Solid Edge part; units mm, degrees
sketch "Sketch1" plane through (0, 0, 0) normal (0, 0, 1) x (1, 0, 0)
  circle A0 centre (0, 0) radius 25.5
extrude "Ajout_matière_1" add sketch "Sketch1" along normal mid plane 71
sketch "Sketch2" plane through (0, 0, 35.5) normal (0, 0, 1) x (1, 0, 0)
  circle A0 centre (0, 0) radius 13
  circle A1 centre (0, 0) radius 5.5
extrude "Ajout_matière_2" add sketch "Sketch2" along normal blind 6
sketch "Sketch3" plane through (0, 0, 35.5) normal (0, 0, 1) x (1, 0, 0)
  circle A0 centre (20.5, 0) radius 2
extrude "Ajout_matière_3" add sketch "Sketch3" along normal blind 10
mirror "Mirror1" about plane through (0, 0, 0) normal (1, 0, 0) of "Ajout_matière_3"
sketch "Sketch4" plane through (0, 0, 35.5) normal (0, 0, 1) x (1, 0, 0)
  circle A0 centre (0, 0) radius 4
extrude "Ajout_matière_5" add sketch "Sketch4" along normal blind 43
cosmetic_thread "Filetage_1" thread depth 13
cosmetic_thread "Thread1"
cosmetic_thread "Thread2"
properties material "Acier S235"
Input: part model. Units: mm. Frame: model coordinates. A direction names the side the tool comes from. Round coordinates to 2 decimals unless told otherwise and drop trailing zeros. Loops run counter-clockwise (first coordinate to the right, second up) from the corner with the lowest first, then second, coordinate; pieces in that order, holes last.
1) Set-up query: faces 1 (the flat face through (20, 0, 45.5)), 2 (the cylindrical face through (18.9, 1.2, 40.4)), 3 (the flat face through (0, 0, 78.5)). Return all of +Z, -Z, +X, -X, +Y, -Y with unobstructed straight access to the full face (end or side cutting, diameter ignored); none if empty.
Ans:
face 1: +Z, +X, +Y, -Y
face 2: +Z
face 3: +Z, +X, -X, +Y, -Y
2) Pull-direction query (X, two-part tool) for faces 4 (the flat face through (-21, 0, 45.5)), 5 (the cylindrical face through (-5.5, 24.9, -0.5)), 6 (the cylindrical face through (-18.9, -1.2, 40.4)); classes: released by +X, released by -X, zero draft, split by the parting line, or undercut.
Ans:
face 4: zero draft
face 5: split by the parting line
face 6: undercut
3) Pin query (flat end, axial travel): pin 1 (8 mm diameter, centred on x = -20, z = 18, fed in from +Y); pin 2 (5 mm diameter, centred on x = -5, z = 28.5, fed in from -Y); pin 3 (2 mm diameter, centred on x = 16.5, y = 6.5, fed in from +Z). Return the tip coordinate at first contact, or that it passes through.
Ans:
pin 1: stops at y = 19.86
pin 2: stops at y = -25.38
pin 3: stops at z = 35.5
4) Material intervals for line 1 (Y direction, x = 0, z = 36.75); line 2 (Z direction, x = -11.5, y = 6); line 3 (Z direction, x = 9, y = -19), sorted ascending.
Ans:
line 1: y = -13 to -5.5, -4 to 4, 5.5 to 13
line 2: z = -35.5 to 41.5
line 3: z = -35.5 to 35.5
5) Section query D-D on z = 56. Return the cut outline in (x, y).
Ans:
outline: circle Ø8 at (0, 0)
6) Section query A-A on z = 39. Return the cut outline in (x, y), plus the area to 3 significant figures.
Ans:
outline: circle Ø4 at (-20.5, 0); circle Ø26 at (0, 0); circle Ø8 at (0, 0); circle Ø4 at (20.5, 0); hole circle Ø11 at (0, 0)
area: 511 mm2
7) Section query B-B on y = 0. Return the cut outline in (x, z).
Ans:
outline: (-25.5, -35.5) - (25.5, -35.5) - (25.5, 35.5) - (22.5, 35.5) - (22.5, 45.5) - (18.5, 45.5) - (18.5, 35.5) - (13, 35.5) - (13, 41.5) - (5.5, 41.5) - (5.5, 35.5) - (4, 35.5) - (4, 78.5) - (-4, 78.5) - (-4, 35.5) - (-5.5, 35.5) - (-5.5, 41.5) - (-13, 41.5) - (-13, 35.5) - (-18.5, 35.5) - (-18.5, 45.5) - (-22.5, 45.5) - (-22.5, 35.5) - (-25.5, 35.5) - close
8) Section query C-C on x = 0. Return the cut outline in (y, z), plus the area to 4 significant figures.
Ans:
outline: (-25.5, -35.5) - (25.5, -35.5) - (25.5, 35.5) - (13, 35.5) - (13, 41.5) - (5.5, 41.5) - (5.5, 35.5) - (4, 35.5) - (4, 78.5) - (-4, 78.5) - (-4, 35.5) - (-5.5, 35.5) - (-5.5, 41.5) - (-13, 41.5) - (-13, 35.5) - (-25.5, 35.5) - close
area: 4,055 mm2
